from build123d import *

# Parameters (mm, degrees)
SKETCH1_W      = 35
SKETCH1_H      = 35
SKETCH1_R      = 1.8
EXTRUDE1_DEPTH = 1
CHAMFER1_SIZE  = 3


with BuildPart() as part:
    # Sketch1 → Extrude1 (new body)
    with BuildSketch(Plane.XY):
        Rectangle(SKETCH1_W, SKETCH1_H)
        with Locations((-12.75, 12.75)):
            Circle(SKETCH1_R, mode=Mode.SUBTRACT)
        with Locations((12.75, 12.75)):
            Circle(SKETCH1_R, mode=Mode.SUBTRACT)
        with Locations((-12.75, -12.75)):
            Circle(SKETCH1_R, mode=Mode.SUBTRACT)
        with Locations((12.75, -12.75)):
            Circle(SKETCH1_R, mode=Mode.SUBTRACT)
    extrude(amount=EXTRUDE1_DEPTH)

    # Chamfer1
    chamfer1_edges = [part.edges().sort_by_distance(p)[0] for p in [
        (-17.5, 17.5, 0.5),
        (17.5, 17.5, 0.5),
        (17.5, -17.5, 0.5),
        (-17.5, -17.5, 0.5),
    ]]
    chamfer(chamfer1_edges, length=CHAMFER1_SIZE)


solid = part.part
The listing builds one solid part. Answer for the finished solid, in the listing's coordinates (mm). Round coordinates to 2 decimals unless told otherwise and drop trailing zeros. Write each loop counter-clockwise with the first axis right and the second up, starting at its lowest first coordinate (ties: lowest second). Pieces come first, ordered by that corner, then holes. Notation, with made-up numbers: (81.5, -19.75) - (88.5, -19.75) arc R36 cw to (88.5, 19.25) - close; hole circle Ø9 at (-36.75, -7). An arc over 180 degrees is marked (long way). Use one line per item in the form item = value. Start each with the question number.
Item 1: A flat-ended cylindrical pin translates along its axis: pin 1 Ø3 at (x, y) = (-12.75, 12.75) entering from -Z. Find the tip coordinate at first contact, or state that the pin passes through.
Item 2: Determine the mould class of faces 1 (the flat face through (-16, -16, 0.5)), 2 (the flat face through (-0.2, -17.5, 0.5)), 3 (the cylindrical face through (-14.077, 13.967, 0.493)) for opening direction X: +X half, -X half, draft (parallel to the pull), parting line (faces both ways), or undercut.
Item 3: Find the intervals of material crossed by line 1 (Y direction, x = 12.75, z = 0.7); line 2 (Y direction, x = -14, z = 0.3), in increasing order. Write a range as [from, to].
Item 4: A cutting plane is placed at A-A (y = -12.75). Write down the section's boundary in (x, z), plus the area to 3 significant figures.
Item 5: A cutting plane is placed at C-C (z = 0.3). Write down the section's boundary in (x, y), plus the area to 3 significant figures.
Item 6: A cutting plane is placed at D-D (x = -15). Write down the section's boundary in (y, z), plus the area to 3 significant figures.
The answers:
q1.pin_1 = through
q2.face_1 = -X half
q2.face_2 = draft
q2.face_3 = undercut
q3.line_1 = [-17.5, -14.55], [-10.95, 10.95], [14.55, 17.5]
q3.line_2 = [-17.5, -14.05], [-11.45, 11.45], [14.05, 17.5]
q4.outline = (-17.5, 0) - (-14.55, 0) - (-14.55, 1) - (-17.5, 1) - close; (-10.95, 0) - (10.95, 0) - (10.95, 1) - (-10.95, 1) - close; (14.55, 0) - (17.5, 0) - (17.5, 1) - (14.55, 1) - close
q4.area = 27.8 mm^2
q5.outline = (-17.5, -14.5) - (-14.5, -17.5) - (14.5, -17.5) - (17.5, -14.5) - (17.5, 14.5) - (14.5, 17.5) - (-14.5, 17.5) - (-17.5, 14.5) - close; hole circle Ø3.6 at (-12.75, -12.75); hole circle Ø3.6 at (-12.75, 12.75); hole circle Ø3.6 at (12.75, -12.75); hole circle Ø3.6 at (12.75, 12.75)
q5.area = 1,170 mm^2
q6.outline = (-17, 0) - (17, 0) - (17, 1) - (-17, 1) - close
q6.area = 34.0 mm^2
